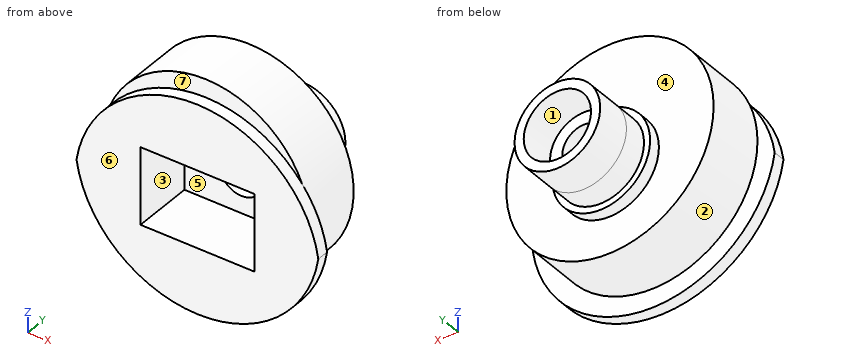
```python
from build123d import *

# Parameters (mm, degrees)
SKETCH1_R           = 3.5
SKETCH1_R_2         = 2.75
BOSS_EXTRUDE1_DEPTH = 3
SKETCH2_R           = 3.5
SKETCH2_R_2         = 1.75
BOSS_EXTRUDE2_DEPTH = 2
SKETCH3_R           = 4
SKETCH3_R_2         = 1.75
BOSS_EXTRUDE3_DEPTH = 1
SKETCH4_R           = 8.475
SKETCH4_R_2         = 1.75
BOSS_EXTRUDE4_DEPTH = 5
SKETCH5_R           = 1.75
BOSS_EXTRUDE5_DEPTH = 1
SKETCH6_W           = 9.3
SKETCH6_H           = 6.3
CUT_EXTRUDE1_DEPTH  = 5


with BuildPart() as part:
    # Sketch1 → Boss-Extrude1 (new body)
    with BuildSketch(Plane(origin=(0, 0, 0), x_dir=(1, 0, 0), z_dir=(0, 1, 0))):
        Circle(SKETCH1_R)
        Circle(SKETCH1_R_2, mode=Mode.SUBTRACT)
    extrude(amount=BOSS_EXTRUDE1_DEPTH)

    # Sketch2 → Boss-Extrude2 (add)
    with BuildSketch(Plane(origin=(0, 0, 0), x_dir=(-1, 0, 0), z_dir=(0, -1, 0))):
        Circle(SKETCH2_R)
        Circle(SKETCH2_R_2, mode=Mode.SUBTRACT)
    extrude(amount=BOSS_EXTRUDE2_DEPTH)

    # Sketch3 → Boss-Extrude3 (add)
    with BuildSketch(Plane(origin=(0, -2, 0), x_dir=(-1, 0, 0), z_dir=(0, -1, 0))):
        Circle(SKETCH3_R)
        Circle(SKETCH3_R_2, mode=Mode.SUBTRACT)
    extrude(amount=BOSS_EXTRUDE3_DEPTH)

    # Sketch4 → Boss-Extrude4 (add)
    with BuildSketch(Plane(origin=(0, -3, 0), x_dir=(-1, 0, 0), z_dir=(0, -1, 0))):
        with Locations((0, -1.5)):
            Circle(SKETCH4_R)
        Circle(SKETCH4_R_2, mode=Mode.SUBTRACT)
    extrude(amount=BOSS_EXTRUDE4_DEPTH)

    # Sketch5 → Boss-Extrude5 (add)
    with BuildSketch(Plane(origin=(0, -8, 0), x_dir=(-1, 0, 0), z_dir=(0, -1, 0))):
        with BuildLine():
            ThreePointArc((-9.886859967, 0), (0, -8.5), (9.886859967, 0))
            ThreePointArc((9.886859967, 0), (0, 8.5), (-9.886859967, 0))
        make_face()
        Circle(SKETCH5_R, mode=Mode.SUBTRACT)
    extrude(amount=BOSS_EXTRUDE5_DEPTH)

    # Sketch6 → Cut-Extrude1 (cut)
    with BuildSketch(Plane(origin=(0, -9, 0), x_dir=(-1, 0, 0), z_dir=(0, -1, 0))):
        Rectangle(SKETCH6_W, SKETCH6_H)
    extrude(amount=-CUT_EXTRUDE1_DEPTH, mode=Mode.SUBTRACT)


solid = part.part
```
Here's how the part is built. I have some questions about the finished solid (model axes, mm). Face numbers are marked on the shaded views. A direction names the side the tool comes from. Give positions to 0.01 mm unless a question says otherwise; leave off trailing zeros. Write each loop counter-clockwise with the first axis right and the second up, starting at its lowest first coordinate (ties: lowest second). Pieces come first, ordered by that corner, then holes.
(1) Imagine slicing it at D-D, the plane x = 3. Write out the boundary of the cut face in (y, z), and give its area (3 significant figures).
Output values:
outline: (-9, -8.04) - (-8, -8.04) - (-8, -6.43) - (-3, -6.43) - (-3, -2.65) - (-2, -2.65) - (-2, -1.8) - (3, -1.8) - (3, 1.8) - (-2, 1.8) - (-2, 2.65) - (-3, 2.65) - (-3, 9.43) - (-8, 9.43) - (-8, 8.04) - (-9, 8.04) - (-9, 3.15) - (-4, 3.15) - (-4, -3.15) - (-9, -3.15) - close
area: 87.2 mm2
(2) If I drill on L1, parallel to X at y = 1.6, z = 0; L2, parallel to Z at x = -1, y = -5.75, over which ranges is the centre line in solid material (lowest first)?
Output values:
L1: x = -3.5 to -2.75, 2.75 to 3.5
L2: z = -6.92 to -3.15, 3.15 to 9.92
(3) On a 3-axis mill with a long thin cutter (end or side, diameter ignored), from which of +Z, -Z, +X, -X, +Y, -Y can I reach the whole of each face in a straight line? I mean the marked faces 5, 6 and 7. Say none if no direction works.
Output values:
face 5: -Y
face 6: +Z, -Z, +X, -X, -Y
face 7: +Z, -Y
(4) Imagine slicing it at A-A, the plane x = 0. Write out the boundary of the cut face in (y, z) (3 decimals), and give its area (4 significant figures).
Output values:
outline: (-9, -8.5) - (-8, -8.5) - (-8, -6.975) - (-3, -6.975) - (-3, -4) - (-2, -4) - (-2, -3.5) - (3, -3.5) - (3, -2.75) - (0, -2.75) - (0, -1.75) - (-4, -1.75) - (-4, -3.15) - (-9, -3.15) - close; (-9, 3.15) - (-4, 3.15) - (-4, 1.75) - (0, 1.75) - (0, 2.75) - (3, 2.75) - (3, 3.5) - (-2, 3.5) - (-2, 4) - (-3, 4) - (-3, 9.975) - (-8, 9.975) - (-8, 8.5) - (-9, 8.5) - close
area: 82.75 mm2
(5) Thinking about a two-plate mould opening in Z: for the marked faces 1, 2, 3 and 4, which applies, pulls with the +Z half, pulls with the -Z half, needs draft (parallel to the pull), parting line crosses it, or undercut?
Output values:
face 1: undercut
face 2: parting line crosses it
face 3: undercut
face 4: needs draft
(6) Will these pins go through, and if not, where does the flat tip stop? pin 1 (1.5 mm diameter, centred on y = -6, z = 1, fed in from +X) (3 decimals); pin 2 (2 mm diameter, centred on y = -3.5, z = 7.5, fed in from +X); pin 3 (3 mm diameter, centred on x = -1, z = 0, fed in from +Y).
Output values:
pin 1: stops at x = 8.475
pin 2: stops at x = 6.84
pin 3: stops at y = 0
(7) Imagine slicing it at C-C, the plane z = 1.5. Write out the boundary of the cut face in (x, y) (3 decimals), and give its area (3 significant figures).
Output values:
outline: (-9.539, -9) - (-4.65, -9) - (-4.65, -4) - (-0.901, -4) - (-0.901, 0) - (-2.305, 0) - (-2.305, 3) - (-3.162, 3) - (-3.162, -2) - (-3.708, -2) - (-3.708, -3) - (-8.475, -3) - (-8.475, -8) - (-9.539, -8) - close; (0.901, -4) - (4.65, -4) - (4.65, -9) - (9.539, -9) - (9.539, -8) - (8.475, -8) - (8.475, -3) - (3.708, -3) - (3.708, -2) - (3.162, -2) - (3.162, 3) - (2.305, 3) - (2.305, 0) - (0.901, 0) - close
area: 75.3 mm2
(8) Imagine slicing it at B-B, the plane y = -6.25. Write out the boundary of the cut face in (x, z) (3 decimals).
Output values:
outline: circle Ø16.95 at (0, 1.5); hole (-4.65, -3.15) - (4.65, -3.15) - (4.65, 3.15) - (-4.65, 3.15) - close
